```python
from build123d import *

# Parameters (mm, degrees)
SKETCH1_R           = 127
SKETCH1_R_2         = 123.825
BOSS_EXTRUDE1_DEPTH = 416.052
SKETCH1_3_R         = 139.7
SKETCH1_3_R_2       = 127
BOSS_EXTRUDE2_DEPTH = 12.7
BOSS_EXTRUDE4_START = 403.352
SKETCH1_5_R         = 139.7
SKETCH1_5_R_2       = 127
BOSS_EXTRUDE4_DEPTH = 12.7


with BuildPart() as part:
    # Sketch1 → Boss-Extrude1 (new body)
    with BuildSketch(Plane(origin=(0, 0, 0), x_dir=(1, 0, 0), z_dir=(0, 1, 0))):
        with Locations(Location((0, 0, 0), (0, 0, 270))):
            Circle(SKETCH1_R)
        with Locations(Location((0, 0, 0), (0, 0, 270))):
            Circle(SKETCH1_R_2, mode=Mode.SUBTRACT)
    extrude(amount=BOSS_EXTRUDE1_DEPTH)

    # Sketch1_3 → Boss-Extrude2 (add)
    with BuildSketch(Plane(origin=(0, 0, 0), x_dir=(1, 0, 0), z_dir=(0, 1, 0))):
        with Locations(Location((0, 0, 0), (0, 0, 270))):
            Circle(SKETCH1_3_R)
        with Locations(Location((0, 0, 0), (0, 0, 270))):
            Circle(SKETCH1_3_R_2, mode=Mode.SUBTRACT)
    extrude(amount=BOSS_EXTRUDE2_DEPTH)

    # Sketch1_5 → Boss-Extrude4 (add)
    with BuildSketch(Plane(origin=(0, 0, 0), x_dir=(1, 0, 0), z_dir=(0, 1, 0)).offset(BOSS_EXTRUDE4_START)):
        with Locations(Location((0, 0, 0), (0, 0, 270))):
            Circle(SKETCH1_5_R)
        with Locations(Location((0, 0, 0), (0, 0, 270))):
            Circle(SKETCH1_5_R_2, mode=Mode.SUBTRACT)
    extrude(amount=BOSS_EXTRUDE4_DEPTH)


solid = part.part
```
Input: part model. Units: mm. Frame: model coordinates. A direction names the side the tool comes from. Round coordinates to 2 decimals unless told otherwise and drop trailing zeros. Write each loop counter-clockwise with the first axis right and the second up, starting at its lowest first coordinate (ties: lowest second). Pieces come first, ordered by that corner, then holes. Notation, with made-up numbers: M 5,83 L 19,83 A21 cw 19,113 Z; hole C 71.25,23 d8. An arc over 180 degrees is marked long. Write each question's results on one line, items separated by ' | '.
Q1. Section query B-B (z = 0). Return loops of the section in (x, y) (3 decimals).
Results:
outline: M -139.7,0 L -123.825,0 L -123.825,416.052 L -139.7,416.052 L -139.7,403.352 L -127,403.352 L -127,12.7 L -139.7,12.7 Z; M 123.825,0 L 139.7,0 L 139.7,12.7 L 127,12.7 L 127,403.352 L 139.7,403.352 L 139.7,416.052 L 123.825,416.052 Z
Q2. Access query for faces 4 (the face through (-136.38, 6.26, -30.28)), 5 (the face through (-124, 403.352, 30)). Directions: +Z, -Z, +X, -X, +Y, -Y. A direction counts if a zero-diameter tool reaches every point of the face in a straight line with its end or side. Return the directions, or none.
Results:
face 4: +Y, -Y | face 5: none
Q3. Line query: line 1 along X through (y, z) = (298.5, 0) (3 decimals); line 2 along Y through (x, z) = (78, 104.5); line 3 along Z through (x, y) = (4, 239). Output: solid intervals per line, ascending.
Results:
line 1: x = -127 to -123.825, 123.825 to 127 | line 2: y = 0 to 12.7, 403.35 to 416.05 | line 3: z = -126.94 to -123.76, 123.76 to 126.94
Q4. Section query A-A (x = 0). Return loops of the section in (y, z) (3 decimals), and give its area (3 significant figures).
Results:
outline: M 0,-139.7 L 12.7,-139.7 L 12.7,-127 L 403.352,-127 L 403.352,-139.7 L 416.052,-139.7 L 416.052,-123.825 L 0,-123.825 Z; M 0,123.825 L 416.052,123.825 L 416.052,139.7 L 403.352,139.7 L 403.352,127 L 12.7,127 L 12.7,139.7 L 0,139.7 Z | area: 3,290 mm^2
Q5. Draft query along X for faces 1 (the face through (-124, 416.052, -11)), 2 (the face through (-120.88, 205.11, -26.84)), 3 (the face through (-123.98, 205.29, -27.53)). Return one class per face: released by +X, released by -X, zero draft, split by the parting line, or undercut.
Results:
face 1: zero draft | face 2: undercut | face 3: split by the parting line
Q6. Section query C-C (y = 340.5). Return loops of the section in (x, z) (3 decimals), and give its area (3 significant figures).
Results:
outline: C 0,0 d254; hole C 0,0 d247.65 | area: 2,500 mm^2
Q7. Pin query (flat end, axial travel): P1, Ø3, axis at x = 84.5, y = 318.5, coming from the +Z side; P2, Ø3, axis at y = 172, z = -44, coming from the -X side; P3, Ø2, axis at x = -41, y = 67.5, coming from the +Z side. Return the tip coordinate at first contact, or that it passes through.
Results:
P1: stops at z = 96.12 | P2: stops at x = -119.68 | P3: stops at z = 120.54
